Verification items for the finished model (mm, model axes). Coordinates: 2 decimals unless noted, no trailing zeros. Order: outer loops, then holes, each group sorted by start corner. A loop starts at its lowest first (then second) coordinate and runs counter-clockwise, first axis right, second up. Notation, with made-up numbers: M 71,33.25 L 94,33.25 A20 cw 94,43.25 Z; hole C 59.25,22.5 d11. An arc over 180 degrees is marked long. Return JSON: item names as keys, results as strings. Group by question number.
1. Section check A-A, the plane x = 0. Record the cut outline in (y, z), plus the area to 3 significant figures.
2. Section check B-B, the plane y = 6. Record the cut outline in (x, z), plus the area to 3 significant figures.
3. Section check C-C, the plane y = 18.5. Record the cut outline in (x, z), plus the area to 3 significant figures.
4. Gauge pin test, flat ends, axial feed: pin 1 (4 mm diameter, centred on x = 0, z = 0, fed in from +Y); pin 2 (6 mm diameter, centred on y = 18, z = 39, fed in from +X); pin 3 (3 mm diameter, centred on x = 38.5, y = 12, fed in from -Z); pin 4 (1 mm diameter, centred on x = -24, y = 18, fed in from -Z). Record the tip position at first contact, or that the pin passes through.
5. Material ranges on line 1 along X through (y, z) = (20.5, 0); line 2 along Z through (x, y) = (44.5, 10); line 3 along Z through (x, y) = (12, 16.75), recorded low to high.
6. Section check D-D, the plane z = -35. Record the cut outline in (x, y), plus the area to 3 significant figures.
```python
from build123d import *
from build123d.topology import SkipClean

# Parameters (mm, degrees)
ESQUISSE1_R             = 50
BOSS_EXTRU_1_DEPTH      = 22
ESQUISSE4_R             = 2.5
ENL_V_MAT_EXTRU_1_DEPTH = 7
ENL_V_START             = -15
ENL_V_MAT_EXTRU_2_DEPTH = 15


with BuildPart() as part:
    # Esquisse1 → Boss.-Extru.1 (new body)
    with BuildSketch(Plane(origin=(0, 0, 0), x_dir=(1, 0, 0), z_dir=(0, 1, 0))):
        with Locations(Location((0, 0, 0), (0, 0, 270))):
            Circle(ESQUISSE1_R)
    extrude(amount=BOSS_EXTRU_1_DEPTH)

    # Esquisse4 → Enlèv. mat.-Extru.1 (cut)
    with BuildSketch(Plane(origin=(0, 22, 0), x_dir=(1, 0, 0), z_dir=(0, 1, 0))):
        with Locations(Location((0, 0, 0), (0, 0, 270))):
            Circle(ESQUISSE4_R)
    extrude(amount=-ENL_V_MAT_EXTRU_1_DEPTH, mode=Mode.SUBTRACT)

    # Esquisse5 → Enlèv. mat.-Extru.2 (cut)
    with SkipClean():  # the faces are left unmerged after this step: merging them gives an invalid solid
        with BuildSketch(Plane(origin=(0, 0, 0), x_dir=(-1, 0, 0), z_dir=(0, -1, 0)).offset(ENL_V_START)):
            with BuildLine():
                ThreePointArc((2.5, 0), (-2.278226738, 1.02940902), (1.652253656, -1.876181723))
                Line((1.652253656, -1.876181723), (2.493901331, -0.174516908))
                ThreePointArc((2.493901331, -0.174516908), (2.498474868, -0.087311719), (2.5, 0))
            make_face()
        extrude(amount=ENL_V_MAT_EXTRU_2_DEPTH, mode=Mode.SUBTRACT)


solid = part.part
```
Answers follow:
{
 "1": {"outline": "M 0,-50 L 22,-50 L 22,-2.5 L 0,-2.5 Z; M 0,2.5 L 22,2.5 L 22,50 L 0,50 Z", "area": "2,090 mm^2"},
 "2": {"outline": "C 0,0 d100; hole M -2.49,0.17 A2.5 ccw long -1.65,1.88 Z", "area": "7,830 mm^2"},
 "3": {"outline": "C 0,0 d100; hole C 0,0 d5", "area": "7,830 mm^2"},
 "4": {"pin 1": "through", "pin 2": "x = 34.7", "pin 3": "z = -33.63", "pin 4": "z = -44.13"},
 "5": {"line 1": "-50 to -2.5, 2.5 to 50", "line 2": "-22.8 to 22.8", "line 3": "-48.54 to 48.54"},
 "6": {"outline": "M -35.71,0 L 35.71,0 L 35.71,22 L -35.71,22 Z", "area": "1,570 mm^2"}
}
